Check sheet for the modelled part. Datum: model origin and axes. Units: mm. Give positions to 0.01 mm unless a question says otherwise; leave off trailing zeros. Loops run counter-clockwise (first coordinate to the right, second up) from the corner with the lowest first, then second, coordinate; pieces in that order, holes last. Notation, with made-up numbers: (66.5, 70) -> (88.5, 70) arc R20 cw to (88.5, 79) -> close; hole circle Ø8 at (-22, 42). An arc over 180 degrees is marked (long way). Answer as CSV lines item,"result". Start each with the question number.
(1) Section check D-D on y = 3.75. Enter the section's corners in (x, z).
(2) Section check B-B on z = 0.55. Enter the section's corners in (x, y), plus the area to 3 significant figures.
(3) Material ranges on line 1 (X direction, y = 0, z = 1.45); line 2 (Y direction, x = -7.5, z = 0.75); line 3 (X direction, y = -1.5, z = 1.35) (3 decimals), recorded low to high. Write a range as from..to.
(4) Section check A-A on x = -18. Enter the section's corners in (y, z), plus the area to 3 significant figures.
(5) Section check C-C on x = 16.5. Enter the section's corners in (y, z) (3 decimals), plus the area to 3 significant figures.
Autodesk Fusion 360 part; units mm, degrees
sketch "Sketch1" plane through (0, 0, 0) normal (0, 0, 1) x (1, 0, 0)
  line L0 (22.5, 4.5) -> (-22.5, 4.5)
  line L1 (-22.5, 4.5) -> (-22.5, -4.5)
  line L2 (-22.5, -4.5) -> (22.5, -4.5)
  line L3 (22.5, -4.5) -> (22.5, 4.5)
  line L4 (22.5, 4.5) -> (-22.5, -4.5) construction
  line L5 (-22.5, 4.5) -> (22.5, -4.5) construction
  dimension "d1" = 45
  dimension "d2" = 9
extrude "Extrude1" add sketch "Sketch1" along normal blind 2
fillet "Fillet1" radius 2.5 4 edges at (-22.5, 4.5, 1) (-22.5, -4.5, 1) (22.5, -4.5, 1) (22.5, 4.5, 1)
sketch "Sketch2" plane through (0, 0, 2) normal (0, 0, 1) x (-1, 0, 0)
  arc A0 (-22.5, -2) -> (-20, -4.5) centre (-20, -2) ccw
  line L0 (-20, -4.5) -> (20, -4.5)
  arc A1 (22.5, 2) -> (20, 4.5) centre (20, 2) ccw
  line L1 (20, 4.5) -> (-20, 4.5)
  arc A2 (20, -4.5) -> (22.5, -2) centre (20, -2) ccw
  line L2 (22.5, -2) -> (22.5, 2)
  arc A3 (-20, 4.5) -> (-22.5, 2) centre (-20, 2) ccw
  line L3 (-22.5, 2) -> (-22.5, -2)
  line L4 (22.5, 0) -> (-22.5, 0) construction
  line L5 (22.5, 0) -> (18, 0)
  line L6 (-22.5, 0) -> (-18, 0)
  circle A4 centre (18, 0) radius 2.7
  circle A5 centre (-18, 0) radius 2.7
  dimension "d15" = 4.5
  dimension "d16" = 4.5
  dimension "d17" = 5.4
  dimension "d18" = 5.4
extrude "Extrude2" cut sketch "Sketch2" against normal blind 3 contours A4 | A5
sketch "Sketch3" plane through (0, 0, 2) normal (0, 0, 1) x (-1, 0, 0)
  arc A0 (-22.5, -2) -> (-20, -4.5) centre (-20, -2) ccw
  line L0 (-20, -4.5) -> (20, -4.5)
  arc A1 (22.5, 2) -> (20, 4.5) centre (20, 2) ccw
  line L1 (20, 4.5) -> (-20, 4.5)
  arc A2 (20, -4.5) -> (22.5, -2) centre (20, -2) ccw
  line L2 (22.5, -2) -> (22.5, 2)
  arc A3 (-20, 4.5) -> (-22.5, 2) centre (-20, 2) ccw
  line L3 (-22.5, 2) -> (-22.5, -2)
  circle A4 centre (18, 0) radius 2.7
  circle A5 centre (-18, 0) radius 2.7
  line L4 (22.5, 0) -> (-22.5, 0) construction
  line L5 (22.5, 0) -> (7.5, 0)
  circle A6 centre (7.5, 0) radius 2.7
  dimension "d19" = 15
  dimension "d20" = 5.4
extrude "Extrude3" cut sketch "Sketch3" against normal blind 2 contours A6
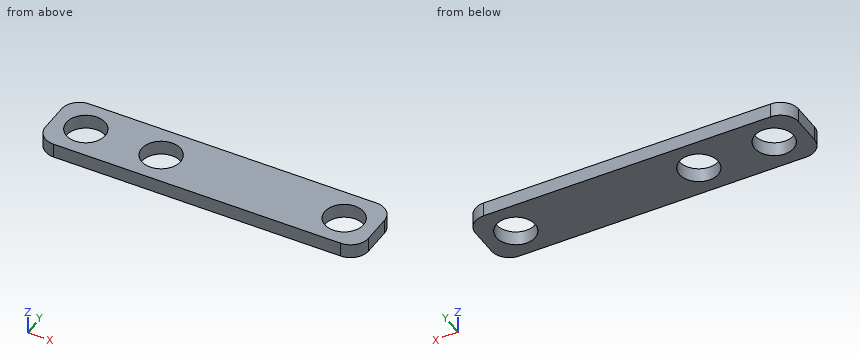
Working result:
1,outline,"(-21.79, 0) -> (21.79, 0) -> (21.79, 2) -> (-21.79, 2) -> close"
2,outline,"(-22.5, -2) arc R2.5 ccw to (-20, -4.5) -> (20, -4.5) arc R2.5 ccw to (22.5, -2) -> (22.5, 2) arc R2.5 ccw to (20, 4.5) -> (-20, 4.5) arc R2.5 ccw to (-22.5, 2) -> close; hole circle Ø5.4 at (-18, 0); hole circle Ø5.4 at (-7.5, 0); hole circle Ø5.4 at (18, 0)"
2,area,"331 mm^2"
3,line 1,"x = -22.5..-20.7, -15.3..-10.2, -4.8..15.3, 20.7..22.5"
3,line 2,"y = -4.5..-2.7, 2.7..4.5"
3,line 3,"x = -22.5..-20.245, -15.755..-9.745, -5.255..15.755, 20.245..22.5"
4,outline,"(-4.5, 0) -> (-2.7, 0) -> (-2.7, 2) -> (-4.5, 2) -> close; (2.7, 0) -> (4.5, 0) -> (4.5, 2) -> (2.7, 2) -> close"
4,area,"7.20 mm^2"
5,outline,"(-4.5, 0) -> (-2.245, 0) -> (-2.245, 2) -> (-4.5, 2) -> close; (2.245, 0) -> (4.5, 0) -> (4.5, 2) -> (2.245, 2) -> close"
5,area,"9.02 mm^2"
